Autodesk Inventor part; units mm, degrees
ref_plane "YZ Plane" through (0, 0, 0) normal (1, 0, 0) x (0, 1, 0)
ref_plane "XZ Plane" through (0, 0, 0) normal (0, 1, 0) x (-1, 0, 0)
ref_plane "XY Plane" through (0, 0, 0) normal (0, 0, 1) x (1, 0, 0)
sketch "Sketch1" plane through (0, 0, 0) normal (0, 0, 1) x (1, 0, 0)
  circle A0 centre (0, 0) radius 6.925
  dimension "d0" = 13.85
extrude "Extrusion1" add sketch "Sketch1" along normal mid plane 153.5
sketch "Sketch2" plane through (0, 0, 76.75) normal (0, 0, 1) x (1, 0, 0)
  circle A0 centre (0, 0) radius 6.925
  point P0 (0, 6.925)
ref_plane "Work Plane1" through (0, 6.925, 76.75) normal (0, 1, 0) x (-1, 0, 0)
sketch "Sketch3" plane through (0, 6.925, 76.75) normal (0, 1, 0) x (-1, 0, 0)
  circle A0 centre (0, -53.585) radius 2.875
  line L0 (6.925, 0) -> (-6.925, 0)
  point P0 (0, -76.75)
  dimension "d3" = 50.71
  dimension "d4" = 5.75
extrude "Extrusion2" add sketch "Sketch3" along normal mid plane 2.92
fillet "Fillet1" radius 1 1 edges at (2.875, 8.385, 23.165)
sketch "Sketch4" plane through (0, 0, 76.75) normal (0, 0, 1) x (1, 0, 0)
  circle A0 centre (0, 0) radius 2.75
  dimension "d8" = 5.5
extrude "Extrusion3" cut sketch "Sketch4" against normal blind 30
fillet "Fillet2" radius 2 2 edges at (-6.925, 0, 76.75) (-6.925, 0, -76.75)
properties part number "Pen_Model"
For this review, take the finished solid that the model builds, in its own axes (mm). A direction names the side the tool comes from. Coordinates: 2 decimals unless noted, no trailing zeros. Loops run counter-clockwise (first coordinate to the right, second up) from the corner with the lowest first, then second, coordinate; pieces in that order, holes last.
1. For line 1 (Y direction, x = 0, z = 60) (3 decimals); line 2 (X direction, y = -0.5, z = 33.5); line 3 (Z direction, x = 2.5, y = 4.5), list the stretches that pass through material, from the lowest coordinate up.
2. Add section B-B, the plane x = 0. Give the boundary of the cut face in (y, z) (3 decimals).
3. Add section A-A, the plane y = 0. Give the boundary of the cut face in (x, z) (3 decimals).
4. Mouldability with a two-part tool opening along Y and no side actions: class faces 1 (the flat face through (2.1, -2.1, 76.75)), 2 (the cylindrical face through (6.6, -2.1, -1)), 3 (the cylindrical face through (-0.596, -2.685, 61.96)), 4 (the flat face through (0, 8.385, 23)) as +Y half, -Y half, draft (parallel to the pull), parting line (faces both ways), or undercut.
5. Insertion check: P1, Ø5, axis at x = -1.5, z = 14.5, coming from the -Y side (3 decimals); P2, Ø4.5, axis at x = 0, y = 0, coming from the +Z side; P3, Ø4, axis at y = 6.5, z = 22.5, coming from the -X side; P4, Ø4, axis at y = 6, z = 10, coming from the +X side. Each pin has a flat end and moves straight along its axis. Give the tip position at first contact, or say it passes through.
6. For faces 5 (the flat face through (0, 0, 46.75)), 6 (the flat face through (0, 0, -76.75)), 7 (the cylindrical face through (2.872, 6.955, 23.039)), list the 3-axis set-ups (+Z, -Z, +X, -X, +Y, -Y) from which the entire face can be reached by the end or side of a thin tool; tool diameter is ignored.
7. Add section C-C, the plane z = 36.5. Give the boundary of the cut face in (x, y) (3 decimals).
Result:
1. line 1: y = -6.925 to -2.75, 2.75 to 6.925
1. line 2: x = -6.91 to 6.91
1. line 3: z = -76.74 to 76.74
2. outline: (-6.925, -74.75) arc R2 ccw to (-4.925, -76.75) - (4.925, -76.75) arc R2 ccw to (6.925, -74.75) - (6.925, 20.29) - (7.385, 20.29) arc R1 ccw to (8.385, 21.29) - (8.385, 25.04) arc R1 ccw to (7.385, 26.04) - (6.925, 26.04) - (6.925, 74.75) arc R2 ccw to (4.925, 76.75) - (2.75, 76.75) - (2.75, 46.75) - (-2.75, 46.75) - (-2.75, 76.75) - (-4.925, 76.75) arc R2 ccw to (-6.925, 74.75) - close
3. outline: (-6.925, -74.75) arc R2 ccw to (-4.925, -76.75) - (4.925, -76.75) arc R2 ccw to (6.925, -74.75) - (6.925, 74.75) arc R2 ccw to (4.925, 76.75) - (2.75, 76.75) - (2.75, 46.75) - (-2.75, 46.75) - (-2.75, 76.75) - (-4.925, 76.75) arc R2 ccw to (-6.925, 74.75) - close
4. face 1: draft
4. face 2: parting line
4. face 3: undercut
4. face 4: +Y half
5. P1: stops at y = -6.925
5. P2: stops at z = 46.75
5. P3: stops at x = -5.26
5. P4: stops at x = 5.65
6. face 5: +Z
6. face 6: -Z, +X, -X, +Y, -Y
6. face 7: +Y
7. outline: circle Ø13.85 at (0, 0)
